For this review, take the finished solid that the model builds, in its own axes (mm). A direction names the side the tool comes from. Round coordinates to 2 decimals unless told otherwise and drop trailing zeros. Order: outer loops, then holes, each group sorted by start corner. A loop starts at its lowest first (then second) coordinate and runs counter-clockwise, first axis right, second up. Notation, with made-up numbers: (82.5, 29) -> (137.5, 29) arc R14 cw to (137.5, 43) -> close; hole circle Ø10 at (26.25, 22). An arc over 180 degrees is marked (long way). Use a Markdown table: item, result. Add a question column.
1) Machinability: for faces 4 (the face through (0, -8, 25)), 5 (the face through (-0.59, -13.54, 54.54)), 6 (the face through (0, -6, 17)), which of the approach directions +Z, -Z, +X, -X, +Y, -Y give a long, thin tool a straight path to every point of the face, cutting with its end or side? Answer none if there is none.
2) Consider section B-B (y = -18). State the section outline as (x, z) points.
3) Draft analysis for pull direction X (two halves, no side actions). For faces 1 (the face through (2, -4, 34)), 2 (the face through (9, -4, 2)), 3 (the face through (-2, -16, 49)), state which applies: pulls with the +X half, pulls with the -X half, needs draft (parallel to the pull), parting line crosses it, or undercut.
4) Consider section A-A (x = 0). Give the number of separate pieces and of enclosed holes in the cut face, plus the area to 3 significant figures.
5) Consider section C-C (z = 13.25). State the section outline as (x, y) points.
6) Consider section D-D (y = -3). State the section outline as (x, z) points.
7) Wall thickness on line 1 along Z through (x, y) = (0, -5.25); line 2 along Z through (x, y) = (0, -2.95); line 3 along Y through (x, z) = (-7, 10): over which ranges is each line inside the solid? List them lowest first. Write a range as [from, to].
8) Clearance check with flat-ended pins moving along their axes: P1, Ø6, axis at x = 5.5, z = 34, coming from the -Y side; P2, Ø2, axis at x = -0.5, y = -19, coming from the +Z side; P3, Ø10, axis at x = -7, y = -24, coming from the -Z side; P4, Ø5.5, axis at x = 0, z = 35.75, coming from the -Y side. State where each tip first meets the part, or that it passes through.
```python
from build123d import *

# Parameters (mm, degrees)
F0_W     = 20
F0_H     = 49
F0_R     = 2.1
F1_DEPTH = 8
F2_R     = 3.75
F3_DEPTH = 4
F4_W     = 20
F4_H     = 8
F5_DEPTH = 28
F6_R     = 2.6
F7_DEPTH = 57.001
F8_R     = 4.5
F9_DEPTH = 5
F10_R    = 5


with BuildPart() as f1:
    # F0 (on Front) → F1 (new body)
    with BuildSketch(Plane.XZ):
        with Locations((0, 24.5)):
            Rectangle(F0_W, F0_H)
        with Locations((0, 13.25)):
            Circle(F0_R, mode=Mode.SUBTRACT)
        with Locations((0, 35.75)):
            Circle(F0_R, mode=Mode.SUBTRACT)
    extrude(amount=F1_DEPTH)

    # F2 (on face) → F3 (cut)
    with BuildSketch(Plane.XZ.offset(8)):
        with Locations((0, 35.75)):
            Circle(F2_R)
        with Locations((0, 13.25)):
            Circle(F2_R)
    extrude(amount=-F3_DEPTH, mode=Mode.SUBTRACT)

    # F4 (on face) → F5 (join)
    with BuildSketch(Plane(origin=(0, 0, 0), x_dir=(-1, 0, 0), z_dir=(0, 1, 0))):
        with Locations((0, 53)):
            Rectangle(F4_W, F4_H)
    extrude(amount=-F5_DEPTH)

    # F6 (on face) → F7 (cut, through all)
    with BuildSketch(Plane.XY.offset(57)):
        with Locations((0, -18)):
            Circle(F6_R)
    extrude(amount=-F7_DEPTH, mode=Mode.SUBTRACT)

    # F8 (on face) → F9 (cut)
    with BuildSketch(Plane.XY.offset(57)):
        with Locations((0, -18)):
            Circle(F8_R)
    extrude(amount=-F9_DEPTH, mode=Mode.SUBTRACT)

    # F10
    f10_edges = [f1.edges().sort_by_distance(p)[0] for p in [
        (10, -28, 53),
        (-10, -28, 53),
        (0, 0, 57),
        (10, -4, 0),
        (-10, -4, 0),
    ]]
    fillet(f10_edges, radius=F10_R)


solid = f1.part
```
Results list:
| question | item | result |
|---|---|---|
| 1 | face 4 | -Z, +X, -X, -Y |
| 1 | face 5 | +Z |
| 1 | face 6 | -Y |
| 2 | outline | (-10, 49) -> (-2.6, 49) -> (-2.6, 52) -> (-4.5, 52) -> (-4.5, 57) -> (-10, 57) -> close; (2.6, 49) -> (10, 49) -> (10, 57) -> (4.5, 57) -> (4.5, 52) -> (2.6, 52) -> close |
| 3 | face 1 | undercut |
| 3 | face 2 | pulls with the +X half |
| 3 | face 3 | needs draft |
| 4 | separate pieces | 4 |
| 4 | enclosed holes | 0 |
| 4 | area | 456 mm2 |
| 5 | outline | (-10, -8) -> (-3.75, -8) -> (-3.75, -4) -> (-2.1, -4) -> (-2.1, 0) -> (-10, 0) -> close; (2.1, -4) -> (3.75, -4) -> (3.75, -8) -> (10, -8) -> (10, 0) -> (2.1, 0) -> close |
| 6 | outline | (-10, 5) arc R5 ccw to (-5, 0) -> (5, 0) arc R5 ccw to (10, 5) -> (10, 56.58) -> (-10, 56.58) -> close; hole circle Ø4.2 at (0, 13.25); hole circle Ø4.2 at (0, 35.75) |
| 7 | line 1 | [0, 9.5], [17, 32], [39.5, 57] |
| 7 | line 2 | [0, 11.15], [15.35, 33.65], [37.85, 56.56] |
| 7 | line 3 | [-8, 0] |
| 8 | P1 | y = -8 |
| 8 | P2 | through |
| 8 | P3 | z = 49 |
| 8 | P4 | y = -4 |
